```python
from build123d import *

# Parameters (mm, degrees)
F0_W     = 85
F0_H     = 30
F0_R     = 4.25
F1_DEPTH = 8.2


with BuildPart() as f1:
    # F0 (on Top) → F1 (new body)
    with BuildSketch(Plane.XY):
        with Locations((1.923828, 2.146574)):
            Rectangle(F0_W, F0_H)
        with Locations((-5.576172, 2.146574)):
            Circle(F0_R, mode=Mode.SUBTRACT)
        with Locations((4.423828, 2.146574)):
            Circle(F0_R, mode=Mode.SUBTRACT)
        with Locations((14.423828, 2.146574)):
            Circle(F0_R, mode=Mode.SUBTRACT)
        with Locations((24.423828, 2.146574)):
            Circle(F0_R, mode=Mode.SUBTRACT)
        with Locations((34.423828, 2.146574)):
            Circle(F0_R, mode=Mode.SUBTRACT)
        Polygon((-34.96525, -1.585525), (-33.502803, 8.411704), (-24.113726, 12.143802), (-16.187095, 5.878672), (-17.649542, -4.118557), (-27.038619, -7.850655), align=None, mode=Mode.SUBTRACT)
    extrude(amount=F1_DEPTH)


solid = f1.part
```
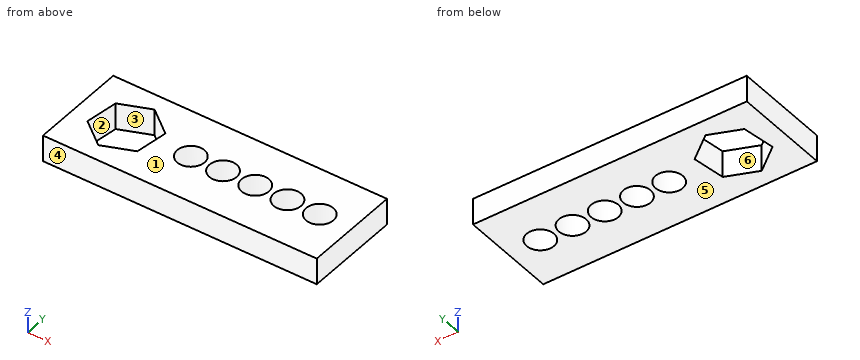
Check sheet for the modelled part. Datum: model origin and axes. Units: mm. Face numbers are marked on the shaded views. A direction names the side the tool comes from. Round coordinates to 2 decimals unless told otherwise and drop trailing zeros. Loops run counter-clockwise (first coordinate to the right, second up) from the corner with the lowest first, then second, coordinate; pieces in that order, holes last. Notation, with made-up numbers: (60, 83.5) -> (107, 83.5) arc R10 ccw to (107, 98.5) -> close; hole circle Ø9 at (49.5, -11.5). An arc over 180 degrees is marked (long way). Write item = value, one per line. Start each with the question number.
1) Sectioned sample at B-B, the plane y = -0.5. Record the cut outline in (x, z).
2) Sectioned sample at D-D, the plane z = 2.5. Record the cut outline in (x, y).
3) Release check for a two-part mould opening along Y. For the marked faces 1, 2, 3 and 4 record: released by +Y, released by -Y, zero draft, split by the parting line, or undercut.
4) Thickness scan on probe 1 along Y at (x, z) = (-18, 4); probe 2 along Y at (x, z) = (4, 3); probe 3 along X at (y, z) = (8, 7). Record the ranges inside material, lowest first.
5) Set-up check for the marked faces 5 and 6: record each of +Z, -Z, +X, -X, +Y, -Y from which the full face is reachable in a straight line by a thin tool's end or side.
6) Gauge pin test, flat end, axial feed: pin 1 Ø5 at (x, y) = (34.42, 2.15) entering from +Z (3 decimals). Record the tip position at first contact, or that the pin passes through.
7) Sectioned sample at A-A, the plane x = -29.5. Record the cut outline in (y, z), plus the area to 3 significant figures.
8) Sectioned sample at C-C, the plane y = 11.25. Record the cut outline in (x, z).
Results are:
q1.outline = (-40.58, 0) -> (-34.81, 0) -> (-34.81, 8.2) -> (-40.58, 8.2) -> close; (-17.12, 0) -> (-8.9, 0) -> (-8.9, 8.2) -> (-17.12, 8.2) -> close; (-2.25, 0) -> (1.1, 0) -> (1.1, 8.2) -> (-2.25, 8.2) -> close; (7.75, 0) -> (11.1, 0) -> (11.1, 8.2) -> (7.75, 8.2) -> close; (17.75, 0) -> (21.1, 0) -> (21.1, 8.2) -> (17.75, 8.2) -> close; (27.75, 0) -> (31.1, 0) -> (31.1, 8.2) -> (27.75, 8.2) -> close; (37.75, 0) -> (44.42, 0) -> (44.42, 8.2) -> (37.75, 8.2) -> close
q2.outline = (-40.58, -12.85) -> (44.42, -12.85) -> (44.42, 17.15) -> (-40.58, 17.15) -> close; hole (-34.97, -1.59) -> (-27.04, -7.85) -> (-17.65, -4.12) -> (-16.19, 5.88) -> (-24.11, 12.14) -> (-33.5, 8.41) -> close; hole circle Ø8.5 at (-5.58, 2.15); hole circle Ø8.5 at (4.42, 2.15); hole circle Ø8.5 at (14.42, 2.15); hole circle Ø8.5 at (24.42, 2.15); hole circle Ø8.5 at (34.42, 2.15)
q3.face_1 = zero draft
q3.face_2 = undercut
q3.face_3 = undercut
q3.face_4 = released by -Y
q4.probe_1 = -12.85 to -4.26, 7.31 to 17.15
q4.probe_2 = -12.85 to -2.08, 6.38 to 17.15
q4.probe_3 = -40.58 to -33.56, -18.87 to 44.42
q5.face_5 = -Z, +X, -X, +Y, -Y
q5.face_6 = +Z, -Z
q6.pin_1 = through
q7.outline = (-12.85, 0) -> (-5.91, 0) -> (-5.91, 8.2) -> (-12.85, 8.2) -> close; (10, 0) -> (17.15, 0) -> (17.15, 8.2) -> (10, 8.2) -> close
q7.area = 116 mm^2
q8.outline = (-40.58, 0) -> (-26.36, 0) -> (-26.36, 8.2) -> (-40.58, 8.2) -> close; (-22.98, 0) -> (44.42, 0) -> (44.42, 8.2) -> (-22.98, 8.2) -> close
